from build123d import *

# Parameters (mm, degrees)
CUT_EXTRUDE1_DEPTH = 1.2
SKETCH5_R          = 1.154700538
CUT_EXTRUDE2_DEPTH = 0.2


with BuildPart() as part:
    # Sketch2 → Revolve1 (revolve)
    with BuildSketch(Plane(origin=(0, 0, 0), x_dir=(0, 0, -1), z_dir=(1, 0, 0))):
        with BuildLine():
            Line((0, 0), (0, 3))
            Line((0, 3), (0.158578644, 3))
            Line((0.158578644, 3), (1.629289322, 1.529289322))
            ThreePointArc((1.629289322, 1.529289322), (1.661731657, 1.507612047), (1.7, 1.5))
            Line((1.7, 1.5), (5.75, 1.5))
            Line((5.75, 1.5), (6, 1.25))
            Line((6, 1.25), (6, 0))
            Line((6, 0), (0, 0))
        make_face()
    revolve(axis=Axis((0, 0, 0), (0, 0, 1)))

    # Sketch3 → Cut-Extrude1 (cut)
    with BuildSketch(Plane.XY):
        Polygon((0, 1.154700538), (-1, 0.577350269), (-1, -0.577350269), (0, -1.154700538), (1, -0.577350269), (1, 0.577350269), align=None)
    extrude(amount=-CUT_EXTRUDE1_DEPTH, mode=Mode.SUBTRACT)

    # Sketch4 → Cut-Revolve1 (revolve, cut)
    with BuildSketch(Plane(origin=(0, 0, 0), x_dir=(0, 0, -1), z_dir=(1, 0, 0))):
        Polygon((1.2, 0), (1.2, 1), (1.777350269, 0), align=None)
    revolve(axis=Axis((0, 0, 0), (0, 0, -1)), mode=Mode.SUBTRACT)

    # Sketch5 → Cut-Extrude2 (cut)
    with BuildSketch(Plane.XY):
        Circle(SKETCH5_R)
    extrude(amount=-CUT_EXTRUDE2_DEPTH, mode=Mode.SUBTRACT)


solid = part.part
Design review of the part built by this model. Coordinates are the model's own, in mm. A direction names the side the tool comes from. Coordinates: 2 decimals unless noted, no trailing zeros. Loops run counter-clockwise (first coordinate to the right, second up) from the corner with the lowest first, then second, coordinate; pieces in that order, holes last. Notation, with made-up numbers: (18, -32.75) - (75, -32.75) arc R12 ccw to (75, -20.75) - close; hole circle Ø10 at (22.25, 43). An arc over 180 degrees is marked (long way). Use CSV: the item, a comma, the result in double quotes. Start each with the question number.
1. To check wall thickness, follow probe 1 along X at (y, z) = (0, -0.1); probe 2 along Y at (x, z) = (0.05, -4.4). State the ranges of each line that lie inside material, in increasing order.
2. Clearance check with flat-ended pins moving along their axes: pin 1 (1 mm diameter, centred on y = 1, z = -3, fed in from +X); pin 2 (0.5 mm diameter, centred on y = 0, z = -0.5, fed in from -X). State where each tip first meets the part, or that it passes through.
3. For faces 1 (the flat face through (-1, 0, -1)), 2 (the flat face through (1, -1, 0)), list the 3-axis set-ups (+Z, -Z, +X, -X, +Y, -Y) from which the entire face can be reached by the end or side of a thin tool; tool diameter is ignored.
4. Add section A-A on z = -3.2. Give the boundary of the cut face in (x, y).
5. Mouldability with a two-part tool opening along X and no side actions: class faces 3 (the cylindrical face through (-0.07, -1.5, -3.75)), 4 (the flat face through (0.51, 0.86, -0.69)), 5 (the flat face through (0, 0, -6)) as released by +X, released by -X, zero draft, split by the parting line, or undercut.
Resolved:
1,probe 1,"-3 to -1.15, 1.15 to 3"
1,probe 2,"-1.5 to 1.5"
2,pin 1,"x = 1.41"
2,pin 2,"x = -2.91"
3,face 1,"+Z"
3,face 2,"+Z, +X, -X, +Y, -Y"
4,outline,"circle Ø3 at (0, 0)"
5,face 3,"split by the parting line"
5,face 4,"undercut"
5,face 5,"zero draft"
